from build123d import *

# Parameters (mm, degrees)
SKETCH1_W           = 70
SKETCH1_H           = 33
BOSS_EXTRUDE1_DEPTH = 35
SKETCH2_W           = 33
SKETCH2_H           = 2
BOSS_EXTRUDE2_DEPTH = 5
SKETCH3_W           = 66
SKETCH3_H           = 29
CUT_EXTRUDE1_DEPTH  = 81.917773835
CUT_EXTRUDE3_DEPTH  = 5
SKETCH13_R          = 2.5
SKETCH13_R_2        = 2.535133393
CUT_EXTRUDE4_DEPTH  = 5
SKETCH14_W          = 33
SKETCH14_H          = 2
BOSS_EXTRUDE4_DEPTH = 5
SKETCH15_R          = 2.5
CUT_EXTRUDE5_DEPTH  = 5
SKETCH17_W          = 80
SKETCH17_H          = 2
BOSS_EXTRUDE6_DEPTH = 5
SKETCH19_W          = 60
SKETCH19_H          = 28.661725901
CUT_EXTRUDE6_DEPTH  = 5
SKETCH20_W          = 60
SKETCH20_H          = 3
CUT_EXTRUDE7_DEPTH  = 5
SKETCH21_W          = 60
SKETCH21_H          = 3
CUT_EXTRUDE8_DEPTH  = 5


with BuildPart() as part:
    # Sketch1 → Boss-Extrude1 (new body)
    with BuildSketch(Plane(origin=(0, 0, 0), x_dir=(1, 0, 0), z_dir=(0, 1, 0))):
        with Locations((-26.152195741, 23.288127357)):
            Rectangle(SKETCH1_W, SKETCH1_H)
    extrude(amount=BOSS_EXTRUDE1_DEPTH)

    # Sketch2 → Boss-Extrude2 (add)
    with BuildSketch(Plane(origin=(8.847804259, 0, 0), x_dir=(0, 0, -1), z_dir=(1, 0, 0))):
        with Locations((23.288127357, 1)):
            Rectangle(SKETCH2_W, SKETCH2_H)
    extrude(amount=BOSS_EXTRUDE2_DEPTH)

    # Sketch3 → Cut-Extrude1 (cut, through all)
    with BuildSketch(Plane(origin=(0, 35, 0), x_dir=(-1, 0, 0), z_dir=(0, 1, 0))):
        with Locations((26.152195741, -23.288127357)):
            Rectangle(SKETCH3_W, SKETCH3_H)
    extrude(amount=-CUT_EXTRUDE1_DEPTH, mode=Mode.SUBTRACT)

    # Sketch9 → Cut-Extrude3 (cut)
    with BuildSketch(Plane.XY.offset(-6.788127357)):
        with BuildLine():
            Line((-27.152195741, 35), (-28.152195741, 35))
            Line((-28.152195741, 35), (-29.152195741, 35))
            ThreePointArc((-29.152195741, 35), (-28.152195741, 34), (-27.152195741, 35))
        make_face()
    extrude(amount=-CUT_EXTRUDE3_DEPTH, mode=Mode.SUBTRACT)

    # Sketch13 → Cut-Extrude4 (cut)
    with BuildSketch(Plane(origin=(8.847804259, 0, 0), x_dir=(0, 0, -1), z_dir=(1, 0, 0))):
        with Locations((13.933834133, 9.111651729)):
            Circle(SKETCH13_R)
        with Locations((13.933834133, 17.855882351)):
            Circle(SKETCH13_R_2)
        with Locations((13.933834133, 26.803467174)):
            Circle(SKETCH13_R)
        with Locations((23.999867059, 26.803467174)):
            Circle(SKETCH13_R)
        with Locations((23.999867059, 17.855882351)):
            Circle(SKETCH13_R)
        with Locations((23.999867059, 9.111651729)):
            Circle(SKETCH13_R)
        with Locations((33.150806082, 9.111651729)):
            Circle(SKETCH13_R)
        with Locations((33.150806082, 17.855882351)):
            Circle(SKETCH13_R)
        with Locations((33.150806082, 26.803467174)):
            Circle(SKETCH13_R)
    extrude(amount=-CUT_EXTRUDE4_DEPTH, mode=Mode.SUBTRACT)

    # Sketch14 → Boss-Extrude4 (add)
    with BuildSketch(Plane.ZY.offset(61.152195741)):
        with Locations((-23.288127357, 1)):
            Rectangle(SKETCH14_W, SKETCH14_H)
    extrude(amount=BOSS_EXTRUDE4_DEPTH)

    # Sketch15 → Cut-Extrude5 (cut)
    with BuildSketch(Plane.ZY.offset(61.152195741)):
        with Locations((-32.467310019, 8.356134386)):
            Circle(SKETCH15_R)
        with Locations((-23.146909162, 8.426743484)):
            Circle(SKETCH15_R)
        with Locations((-13.755899208, 8.426743484)):
            Circle(SKETCH15_R)
        with Locations((-13.755899208, 18.029580731)):
            Circle(SKETCH15_R)
        with Locations((-23.146909162, 18.029580731)):
            Circle(SKETCH15_R)
        with Locations((-32.467310019, 18.029580731)):
            Circle(SKETCH15_R)
        with Locations((-32.467310019, 27.349981588)):
            Circle(SKETCH15_R)
        with Locations((-23.146909162, 27.349981588)):
            Circle(SKETCH15_R)
        with Locations((-13.755899208, 27.349981588)):
            Circle(SKETCH15_R)
    extrude(amount=-CUT_EXTRUDE5_DEPTH, mode=Mode.SUBTRACT)

    # Sketch17 → Boss-Extrude6 (add)
    with BuildSketch(Plane.XY.offset(-6.788127357)):
        with Locations((-26.152195741, 1)):
            Rectangle(SKETCH17_W, SKETCH17_H)
    extrude(amount=BOSS_EXTRUDE6_DEPTH)

    # Sketch19 → Cut-Extrude6 (cut)
    with BuildSketch(Plane(origin=(0, 0, -39.788127357), x_dir=(-1, 0, 0), z_dir=(0, 0, -1))):
        with Locations((26.152195741, 20.66913705)):
            Rectangle(SKETCH19_W, SKETCH19_H)
    extrude(amount=-CUT_EXTRUDE6_DEPTH, mode=Mode.SUBTRACT)

    # Sketch20 → Cut-Extrude7 (cut)
    with BuildSketch(Plane.XY.offset(-6.788127357)):
        with Locations((-26.152195741, 28.5)):
            Rectangle(SKETCH20_W, SKETCH20_H)
    extrude(amount=-CUT_EXTRUDE7_DEPTH, mode=Mode.SUBTRACT)

    # Sketch21 → Cut-Extrude8 (cut)
    with BuildSketch(Plane.XY.offset(-6.788127357)):
        with Locations((-26.152195741, 12.5)):
            Rectangle(SKETCH21_W, SKETCH21_H)
        with Locations((-26.152195741, 20.5)):
            Rectangle(SKETCH21_W, SKETCH21_H)
    extrude(amount=-CUT_EXTRUDE8_DEPTH, mode=Mode.SUBTRACT)


solid = part.part
Model file for the job. Use its own axes, mm. A direction names the side the tool comes from. Give positions to 0.01 mm unless a question says otherwise; leave off trailing zeros. Loops run counter-clockwise (first coordinate to the right, second up) from the corner with the lowest first, then second, coordinate; pieces in that order, holes last.
Item 1: Which spindle directions (+Z, -Z, +X, -X, +Y, -Y) get a long thin tool onto all of the face, cutting with end or side? Do faces 4 (the face through (-26, 6.338, -39)), 5 (the face through (-60.17, 15.59, -14.3)), 6 (the face through (7.862, 27.554, -35.535)), 7 (the face through (3.848, 28, -8)), 8 (the face through (-28.2, 34, -7.8)). Say none if no direction does.
Check values:
face 4: -Z, +Y
face 5: -X
face 6: +X
face 7: +Z, -Z
face 8: +Z, -Z, +Y
Item 2: Slice it at C-C (x = -60). Give the number of separate pieces and of enclosed holes in the cut face, plus the area to 3 significant figures.
Check values:
separate pieces: 1
enclosed holes: 9
area: 988 mm2
Item 3: Slice it at A-A (y = 4). Write the cut outline in (x, z), plus the area to 3 significant figures.
Check values:
outline: (-61.15, -39.79) - (8.85, -39.79) - (8.85, -6.79) - (-61.15, -6.79) - close; hole (-59.15, -37.79) - (6.85, -37.79) - (6.85, -8.79) - (-59.15, -8.79) - close
area: 396 mm2
Item 4: Mould opens along Z. For faces 1 (the face through (-61.152, 18, -19)), 2 (the face through (6.848, 18, -27)), 3 (the face through (-27, 1, -1.788)) say: +Z half, -Z half, draft (parallel to the pull), parting line (faces both ways), or undercut.
Check values:
face 1: draft
face 2: undercut
face 3: +Z half
Item 5: Drop flat-ended pins along their axis: P1, Ø6, axis at y = 26.8, z = -24, coming from the +X side; P2, Ø8, axis at y = 9.11, z = -33.15, coming from the -X side; P3, Ø12, axis at x = -16, z = -6, coming from the -Y side; P4, Ø4, axis at y = 27.35, z = -32.47, coming from the -X side. Give the stop position or say it passes through.
Check values:
P1: stops at x = 8.85
P2: stops at x = -61.15
P3: stops at y = 0
P4: stops at x = 6.85
Item 6: Drill centre lines: line 1 along X through (y, z) = (15.5, -25); line 2 along Z through (x, y) = (7, 8); line 3 along Z through (x, y) = (-51.5, 6). Where is each one in solid material? Low to high.
Check values:
line 1: x = -61.15 to -59.15, 6.85 to 8.85
line 2: z = -39.79 to -35.39, -30.91 to -26.24, -21.76 to -16.17, -11.69 to -6.79
line 3: z = -39.79 to -37.79, -8.79 to -6.79
Item 7: Slice it at B-B (x = -22). Write the cut outline in (y, z).
Check values:
outline: (0, -39.79) - (6.34, -39.79) - (6.34, -37.79) - (0, -37.79) - close; (0, -8.79) - (11, -8.79) - (11, -6.79) - (2, -6.79) - (2, -1.79) - (0, -1.79) - close; (14, -8.79) - (19, -8.79) - (19, -6.79) - (14, -6.79) - close; (22, -8.79) - (27, -8.79) - (27, -6.79) - (22, -6.79) - close; (30, -8.79) - (35, -8.79) - (35, -6.79) - (30, -6.79) - close
